from build123d import *

# Parameters (mm, degrees)
BOSS_EXTRUDE1_DEPTH             = 6.35
CUT_EXTRUDE1_REACH              = 84.103
CUT_EXTRUDE2_REACH              = 84.103
SKETCH3_R                       = 6.25
F_3_0MM_CLEARANCE_DOWEL_HOLE1_D = 3
CIRPATTERN1_COUNT               = 6


with BuildPart() as part:
    # Sketch1 → Boss-Extrude1 (new body)
    with BuildSketch(Plane.XY):
        with BuildLine():
            Line((19.5, 0), (19.5, -79.5))
            Line((19.5, -79.5), (-19.5, -79.5))
            Line((-19.5, -79.5), (-19.5, 0))
            ThreePointArc((-19.5, 0), (0, 19.5), (19.5, 0))
        make_face()
    extrude(amount=BOSS_EXTRUDE1_DEPTH)

    # Sketch2 → Cut-Extrude1 (cut, up to next)
    with BuildSketch(Plane.XY.offset(6.35), mode=Mode.PRIVATE) as cut_extrude1_sk1:
        with BuildLine():
            Line((-14.11, -73.5), (-14.11, -65.5))
            ThreePointArc((-14.11, -65.5), (-11.5, -62.89), (-8.89, -65.5))
            Line((-8.89, -65.5), (-8.89, -73.5))
            ThreePointArc((-8.89, -73.5), (-11.5, -76.11), (-14.11, -73.5))
        make_face()
    cut_extrude1_tool1 = extrude(cut_extrude1_sk1.sketch, amount=-CUT_EXTRUDE1_REACH, mode=Mode.PRIVATE) & part.part
    # Sketch2 → Cut-Extrude1 (cut, up to next)
    with BuildSketch(Plane.XY.offset(6.35), mode=Mode.PRIVATE) as cut_extrude1_sk2:
        with BuildLine():
            Line((-14.11, -53.5), (-14.11, -45.5))
            ThreePointArc((-14.11, -45.5), (-11.5, -42.89), (-8.89, -45.5))
            Line((-8.89, -45.5), (-8.89, -53.5))
            ThreePointArc((-8.89, -53.5), (-11.5, -56.11), (-14.11, -53.5))
        make_face()
    cut_extrude1_tool2 = extrude(cut_extrude1_sk2.sketch, amount=-CUT_EXTRUDE1_REACH, mode=Mode.PRIVATE) & part.part
    # Sketch2 → Cut-Extrude1 (cut, up to next)
    with BuildSketch(Plane.XY.offset(6.35), mode=Mode.PRIVATE) as cut_extrude1_sk3:
        with BuildLine():
            Line((14.11, -73.5), (14.11, -65.5))
            ThreePointArc((14.11, -65.5), (11.5, -62.89), (8.89, -65.5))
            Line((8.89, -65.5), (8.89, -73.5))
            ThreePointArc((8.89, -73.5), (11.5, -76.11), (14.11, -73.5))
        make_face()
    cut_extrude1_tool3 = extrude(cut_extrude1_sk3.sketch, amount=-CUT_EXTRUDE1_REACH, mode=Mode.PRIVATE) & part.part
    # Sketch2 → Cut-Extrude1 (cut, up to next)
    with BuildSketch(Plane.XY.offset(6.35), mode=Mode.PRIVATE) as cut_extrude1_sk4:
        with BuildLine():
            Line((14.11, -53.5), (14.11, -45.5))
            ThreePointArc((14.11, -45.5), (11.5, -42.89), (8.89, -45.5))
            Line((8.89, -45.5), (8.89, -53.5))
            ThreePointArc((8.89, -53.5), (11.5, -56.11), (14.11, -53.5))
        make_face()
    cut_extrude1_tool4 = extrude(cut_extrude1_sk4.sketch, amount=-CUT_EXTRUDE1_REACH, mode=Mode.PRIVATE) & part.part
    add(cut_extrude1_tool1.solids().sort_by_distance((-11.5, -69.5, 6.35))[0], mode=Mode.SUBTRACT)
    add(cut_extrude1_tool2.solids().sort_by_distance((-11.5, -49.5, 6.35))[0], mode=Mode.SUBTRACT)
    add(cut_extrude1_tool3.solids().sort_by_distance((11.5, -69.5, 6.35))[0], mode=Mode.SUBTRACT)
    add(cut_extrude1_tool4.solids().sort_by_distance((11.5, -49.5, 6.35))[0], mode=Mode.SUBTRACT)

    # Sketch3 → Cut-Extrude2 (cut, up to next)
    with BuildSketch(Plane.XY.offset(6.35), mode=Mode.PRIVATE) as cut_extrude2_sk1:
        Circle(SKETCH3_R)
    cut_extrude2_tool1 = extrude(cut_extrude2_sk1.sketch, amount=-CUT_EXTRUDE2_REACH, mode=Mode.PRIVATE) & part.part
    add(cut_extrude2_tool1.solids().sort_by_distance((0, 0, 6.35))[0], mode=Mode.SUBTRACT)

    # Ø3.0mm Clearance Dowel Hole1 (through all)
    with Locations(Plane(origin=(0, 15.5, 6.35), x_dir=(1, 0, 0), z_dir=(0, 0, 1))):
        with Locations((0, 0)):
            f_3_0mm_clearance_dowel_hole1 = Hole(F_3_0MM_CLEARANCE_DOWEL_HOLE1_D / 2)

    # CirPattern1: Ø3.0mm Clearance Dowel Hole1 ×6 about axis
    cirpattern1_axis = Axis((0, 0, 0), (0, 0, 1))
    for i in range(1, CIRPATTERN1_COUNT):
        add(f_3_0mm_clearance_dowel_hole1.rotate(cirpattern1_axis, i * 360 / CIRPATTERN1_COUNT), mode=Mode.SUBTRACT)


solid = part.part
Geometry: final body of the model. Coordinates: model frame, mm. A direction names the side the tool comes from. Round coordinates to 2 decimals unless told otherwise and drop trailing zeros. Loops run counter-clockwise (first coordinate to the right, second up) from the corner with the lowest first, then second, coordinate; pieces in that order, holes last. Notation, with made-up numbers: (53, 88.5) -> (69, 88.5) arc R28 ccw to (69, 109.5) -> close; hole circle Ø7 at (48.5, 22). An arc over 180 degrees is marked (long way). One line per question, with ' | ' between items. Start each with the question number.
1. Line query: line 1 along Y through (x, z) = (0, 1.75); line 2 along X through (y, z) = (-8.5, 5.25); line 3 along X through (y, z) = (-67, 4.5). Output: solid intervals per line, ascending. Write a range as [from, to].
2. Mould query, pull axis Y, two halves, no side actions, for faces 1 (the face through (-11.56, -42.89, 3.22)), 2 (the face through (0, -29, 6.35)), 3 (the face through (-0.429, 19.495, 3.131)). Classes: pulls with the +Y half, pulls with the -Y half, needs draft (parallel to the pull), parting line crosses it, or undercut.
3. Section D-D on x = -10. Output: boundary loops of the cut face in (y, z), and give its area (3 significant figures).
4. Section A-A on y = -15.5. Output: boundary loops of the cut face in (x, z).
5. Section C-C on z = 3.25. Count the separate pieces of the cut face and the enclosed holes in it, and give its area (3 significant figures).
6. Section B-B on x = 5. Output: boundary loops of the cut face in (y, z).
7. Set-up query: faces 4 (the face through (19.5, -39, 3)), 5 (the face through (11.56, -42.89, 3.22)). Return all of +Z, -Z, +X, -X, +Y, -Y with unobstructed straight access to the full face (end or side cutting, diameter ignored); none if empty.
8. Contact query for a flat-ended pin moving along its axis: pin 1 (2 mm diameter, centred on x = 0, z = 2, fed in from +Y). Output: stop coordinate, or through.
Returned:
1) line 1: y = [-79.5, -17], [-14, -6.25], [6.25, 14], [17, 19.5] | line 2: x = [-19.5, -14.72], [-12.12, 12.12], [14.72, 19.5] | line 3: x = [-19.5, -14.11], [-8.89, 8.89], [14.11, 19.5]
2) face 1: undercut | face 2: needs draft | face 3: pulls with the +Y half
3) outline: (-79.5, 0) -> (-75.64, 0) -> (-75.64, 6.35) -> (-79.5, 6.35) -> close; (-63.36, 0) -> (-55.64, 0) -> (-55.64, 6.35) -> (-63.36, 6.35) -> close; (-43.36, 0) -> (16.74, 0) -> (16.74, 6.35) -> (-43.36, 6.35) -> close | area: 455 mm2
4) outline: (-19.5, 0) -> (-1.5, 0) -> (-1.5, 6.35) -> (-19.5, 6.35) -> close; (1.5, 0) -> (19.5, 0) -> (19.5, 6.35) -> (1.5, 6.35) -> close
5) separate pieces: 1 | enclosed holes: 11 | area: 3,280 mm2
6) outline: (-79.5, 0) -> (-3.75, 0) -> (-3.75, 6.35) -> (-79.5, 6.35) -> close; (3.75, 0) -> (18.85, 0) -> (18.85, 6.35) -> (3.75, 6.35) -> close
7) face 4: +Z, -Z, +X, +Y, -Y | face 5: +Z, -Z
8) pin 1: stops at y = 19.5
